```python
from build123d import *

# Parameters (mm, degrees)
SKETCH1_W           = 88.9
SKETCH1_H           = 101.6
BOSS_EXTRUDE1_DEPTH = 2.54
SKETCH2_R           = 1.1303
BOSS_EXTRUDE2_DEPTH = 6.35
SKETCH3_W           = 3.81
SKETCH3_H           = 2.54
CUT_EXTRUDE1_DEPTH  = 2.54
FILLET1_R           = 2.54


with BuildPart() as part:
    # Sketch1 → Boss-Extrude1 (new body)
    with BuildSketch(Plane.XY):
        with Locations((44.45, 50.8)):
            Rectangle(SKETCH1_W, SKETCH1_H)
    extrude(amount=BOSS_EXTRUDE1_DEPTH)

    # Sketch2 → Boss-Extrude2 (add)
    with BuildSketch(Plane.XY.offset(2.54)):
        with Locations((11.43, 87.6046)):
            Circle(SKETCH2_R)
        with Locations((77.47, 87.6046)):
            Circle(SKETCH2_R)
        with Locations((77.47, 11.4046)):
            Circle(SKETCH2_R)
        with Locations((11.43, 11.4046)):
            Circle(SKETCH2_R)
    extrude(amount=BOSS_EXTRUDE2_DEPTH)

    # Sketch3 → Cut-Extrude1 (cut)
    with BuildSketch(Plane.XY.offset(2.54)):
        with Locations((19.05, 15.24)):
            Rectangle(SKETCH3_W, SKETCH3_H)
        with Locations((69.85, 10.16)):
            Rectangle(SKETCH3_W, SKETCH3_H)
        with Locations((69.85, 15.24)):
            Rectangle(SKETCH3_W, SKETCH3_H)
        with Locations((19.05, 10.16)):
            Rectangle(SKETCH3_W, SKETCH3_H)
        with Locations((19.05, 86.36)):
            Rectangle(SKETCH3_W, SKETCH3_H)
        with Locations((19.05, 91.44)):
            Rectangle(SKETCH3_W, SKETCH3_H)
        with Locations((69.85, 86.36)):
            Rectangle(SKETCH3_W, SKETCH3_H)
        with Locations((69.85, 91.44)):
            Rectangle(SKETCH3_W, SKETCH3_H)
    extrude(amount=-CUT_EXTRUDE1_DEPTH, mode=Mode.SUBTRACT)

    # Fillet1
    fillet1_edges = [part.edges().sort_by_distance(p)[0] for p in [
        (0, 101.6, 1.27),
        (88.9, 101.6, 1.27),
        (88.9, 0, 1.27),
        (0, 0, 1.27),
    ]]
    fillet(fillet1_edges, radius=FILLET1_R)


solid = part.part
```
CAD build for the part. Positions are in the model's coordinates, mm. A direction names the side the tool comes from. Give positions to 0.01 mm unless a question says otherwise; leave off trailing zeros. Order: outer loops, then holes, each group sorted by start corner. A loop starts at its lowest first (then second) coordinate and runs counter-clockwise, first axis right, second up. Notation, with made-up numbers: M 37,24 L 94,24 A29 cw 94,61 Z; hole C -1,49 d1. An arc over 180 degrees is marked long. Put each result on its own line as item: value. Start each with the question number.
(1) Saw through at D-D, the plane x = 82.5. Write the cut outline in (y, z), then the cut area to 3 significant figures.
(2) Saw through at B-B, the plane z = 7.25. Write the cut outline in (x, y), then the cut area to 3 significant figures.
(3) Flat gauge pin, fed straight in: pin 1 Ø4 at (x, y) = (48, 65.5) entering from +Z. Where does the tip first touch, or does it go through?
(4) Saw through at A-A, the plane x = 11.43. Write the cut outline in (y, z).
(5) Which spindle directions (+Z, -Z, +X, -X, +Y, -Y) get a long thin tool onto all of the face, cutting with end or side? Do faces 1 (the cylindrical face through (78.514, 87.172, 5.671)), 2 (the flat face through (20.955, 86, 1)), 3 (the flat face through (0, 50, 1)). Say none if no direction does.
(6) Mould opens along Y. For faces 4 (the flat face through (77, 11, 8.89)), 5 (the cylindrical face through (11.185, 86.501, 5.671)), 6 (the cylindrical face through (0.724, 100.836, 1.288)), 7 (the flat face through (67.945, 91, 1)) say: +Y half, -Y half, draft (parallel to the pull), parting line (faces both ways), or undercut.
(7) Saw through at C-C, the plane y = 84. Write the cut outline in (x, z), then the cut area to 3 significant figures.
(8) Drill centre lines: line 1 along X through (y, z) = (15.5, 1.5) (3 decimals); line 2 along Y through (x, z) = (70.5, 2.5); line 3 along Z through (x, y) = (31, 95.5). Where is each one in solid material? Low to high.
Check result:
1. outline: M 0,0 L 101.6,0 L 101.6,2.54 L 0,2.54 Z
1. area: 258 mm2
2. outline: C 11.43,11.4 d2.26; C 11.43,87.6 d2.26; C 77.47,11.4 d2.26; C 77.47,87.6 d2.26
2. area: 16.1 mm2
3. pin 1: stops at z = 2.54
4. outline: M 0,0 L 101.6,0 L 101.6,2.54 L 88.73,2.54 L 88.73,8.89 L 86.47,8.89 L 86.47,2.54 L 12.53,2.54 L 12.53,8.89 L 10.27,8.89 L 10.27,2.54 L 0,2.54 Z
5. face 1: +Z
5. face 2: +Z, -Z
5. face 3: +Z, -Z, -X, +Y, -Y
6. face 4: draft
6. face 5: undercut
6. face 6: +Y half
6. face 7: undercut
7. outline: M 0,0 L 88.9,0 L 88.9,2.54 L 0,2.54 Z
7. area: 226 mm2
8. line 1: x = 0 to 17.145, 20.955 to 67.945, 71.755 to 88.9
8. line 2: y = 0 to 8.89, 11.43 to 13.97, 16.51 to 85.09, 87.63 to 90.17, 92.71 to 101.6
8. line 3: z = 0 to 2.54
